```python
from build123d import *

# Parameters (mm, degrees)
F0_R     = 11.05
F0_R_2   = 1
F0_R_3   = 2
F1_DEPTH = 7


with BuildPart() as f1:
    # F0 (on Top) → F1 (new body)
    with BuildSketch(Plane.XY):
        with BuildLine():
            ThreePointArc((-8.1567643089, 17.1600465037), (0, 14.4299215496), (8.1567643089, 17.1600465037))
            ThreePointArc((8.1567643089, 17.1600465037), (12.1269669824, 21.9351575503), (13.55, 27.9799215496))
            ThreePointArc((13.55, 27.9799215496), (-6.0447639993, 40.106888532), (-8.1567643089, 17.1600465037))
        make_face()
        with Locations((0, 27.9799215496)):
            Circle(F0_R, mode=Mode.SUBTRACT)
        with BuildLine():
            ThreePointArc((37.7813228578, -13.9899607748), (31.7112023358, -2.6915581003), (18.9394183568, -1.5160581476))
            ThreePointArc((18.9394183568, -1.5160581476), (12.4966786365, -7.2149607748), (10.7826540478, -15.6439883561))
            ThreePointArc((10.7826540478, -15.6439883561), (25.0598871658, -27.5146042521), (37.7813228578, -13.9899607748))
        make_face()
        with Locations((24.2313228578, -13.9899607748)):
            Circle(F0_R, mode=Mode.SUBTRACT)
        with BuildLine():
            ThreePointArc((-18.9394183568, -1.5160581476), (-35.9659670791, -20.7649607748), (-10.7826540478, -15.6439883561))
            ThreePointArc((-10.7826540478, -15.6439883561), (-10.7066793805, -14.8185250827), (-10.6813228578, -13.9899607748))
            ThreePointArc((-10.6813228578, -13.9899607748), (-12.9329201833, -6.5100812968), (-18.9394183568, -1.5160581476))
        make_face()
        with Locations((-24.2313228578, -13.9899607748)):
            Circle(F0_R, mode=Mode.SUBTRACT)
        with BuildLine():
            ThreePointArc((4.7600365071, -12.6863924128), (11.1377958922, -7.7169944062), (13.55, 0))
            ThreePointArc((13.55, 0), (13.5004224782, 1.1580556593), (13.352052707, 2.3076369968))
            ThreePointArc((13.352052707, 2.3076369968), (11.7125847278, 6.8130653155), (8.6067198583, 10.4655087445))
            ThreePointArc((8.6067198583, 10.4655087445), (-0.0439952769, 13.549928576), (-8.6744986155, 10.4093983385))
            ThreePointArc((-8.6744986155, 10.4093983385), (-11.7565800048, 6.7368632605), (-13.3667563654, 2.2208836683))
            ThreePointArc((-13.3667563654, 2.2208836683), (-11.7125847278, -6.8130653155), (-4.6775540916, -12.7170353353))
            ThreePointArc((-4.6775540916, -12.7170353353), (0.0439952769, -13.549928576), (4.7600365071, -12.6863924128))
        make_face()
        Circle(F0_R, mode=Mode.SUBTRACT)
        with BuildLine():
            ThreePointArc((-8.7748548257, -16.8523565945), (-7.0337804641, -14.4799478416), (-4.6775540916, -12.7170353353))
            ThreePointArc((-4.6775540916, -12.7170353353), (-11.7125847278, -6.8130653155), (-13.3667563654, 2.2208836683))
            ThreePointArc((-13.3667563654, 2.2208836683), (-16.0640126782, 1.044247953), (-18.9869659815, 0.7036496412))
            ThreePointArc((-18.9869659815, 0.7036496412), (-18.9956424716, -0.4068993604), (-18.9394183568, -1.5160581476))
            ThreePointArc((-18.9394183568, -1.5160581476), (-12.9329201833, -6.5100812968), (-10.6813228578, -13.9899607748))
            ThreePointArc((-10.6813228578, -13.9899607748), (-10.7066793805, -14.8185250827), (-10.7826540478, -15.6439883561))
            ThreePointArc((-10.7826540478, -15.6439883561), (-9.7974015323, -16.2791560965), (-8.7748548257, -16.8523565945))
        make_face()
        with BuildLine():
            ThreePointArc((-8.6744986155, 10.4093983385), (-0.0439952769, 13.549928576), (8.6067198583, 10.4655087445))
            ThreePointArc((8.6067198583, 10.4655087445), (8.9363515943, 13.3897190895), (10.1028614554, 16.0913700602))
            ThreePointArc((10.1028614554, 16.0913700602), (9.1454360529, 16.6541586219), (8.1567643089, 17.1600465037))
            ThreePointArc((8.1567643089, 17.1600465037), (0, 14.4299215496), (-8.1567643089, 17.1600465037))
            ThreePointArc((-8.1567643089, 17.1600465037), (-9.1994619657, 16.6243766663), (-10.2071415116, 16.0254254908))
            ThreePointArc((-10.2071415116, 16.0254254908), (-9.0231124442, 13.3314064874), (-8.6744986155, 10.4093983385))
        make_face()
        with BuildLine():
            ThreePointArc((13.352052707, 2.3076369968), (13.5004224782, 1.1580556593), (13.55, 0))
            ThreePointArc((13.55, 0), (11.1377958922, -7.7169944062), (4.7600365071, -12.6863924128))
            ThreePointArc((4.7600365071, -12.6863924128), (7.1276610839, -14.4339670425), (8.8841045261, -16.7950197013))
            ThreePointArc((8.8841045261, -16.7950197013), (9.8502064187, -16.2472592614), (10.7826540478, -15.6439883561))
            ThreePointArc((10.7826540478, -15.6439883561), (12.4966786365, -7.2149607748), (18.9394183568, -1.5160581476))
            ThreePointArc((18.9394183568, -1.5160581476), (18.9968634979, -0.3452205697), (18.9819963373, 0.8269311037))
            ThreePointArc((18.9819963373, 0.8269311037), (16.0568929083, 1.1485413542), (13.352052707, 2.3076369968))
        make_face()
        with BuildLine():
            ThreePointArc((8.6067198583, 10.4655087445), (11.7125847278, 6.8130653155), (13.352052707, 2.3076369968))
            ThreePointArc((13.352052707, 2.3076369968), (16.0568929083, 1.1485413542), (18.9819963373, 0.8269311037))
            ThreePointArc((18.9819963373, 0.8269311037), (23.4304012279, 2.0634206387), (26.8491945381, 5.1664940737))
            ThreePointArc((26.8491945381, 5.1664940737), (28.2136339107, 8.0652639574), (28.5913217984, 11.246759439))
            ThreePointArc((28.5913217984, 11.246759439), (27.2444210774, 15.8477419457), (23.9108601236, 19.2931088268))
            ThreePointArc((23.9108601236, 19.2931088268), (20.9586164714, 20.5376244184), (17.7643170713, 20.7846324805))
            ThreePointArc((17.7643170713, 20.7846324805), (13.3768238274, 19.3468858147), (10.1028614554, 16.0913700602))
            ThreePointArc((10.1028614554, 16.0913700602), (8.9363515943, 13.3897190895), (8.6067198583, 10.4655087445))
        make_face()
        with BuildLine():
            ThreePointArc((12.9505363993, 11.1563030517), (13.5264237307, 11.5666124247), (13.9367331037, 10.9907250933))
            ThreePointArc((13.9367331037, 10.9907250933), (14.5872544025, 8.309022028), (16.9762482984, 6.9279291798))
            ThreePointArc((16.9762482984, 6.9279291798), (17.4128850212, 6.3717382302), (16.8566940716, 5.9351015075))
            ThreePointArc((16.8566940716, 5.9351015075), (13.7865377349, 7.7099787756), (12.9505363993, 11.1563030517))
        make_face(mode=Mode.SUBTRACT)
        with Locations((18.6004471086, 10.8196494619)):
            Circle(F0_R_2, mode=Mode.SUBTRACT)
        with Locations((23.5651301856, 10.2264193675)):
            Circle(F0_R_3, mode=Mode.SUBTRACT)
        with Locations((20.539148591, 15.4284927617)):
            Circle(F0_R_3, mode=Mode.SUBTRACT)
        with BuildLine():
            ThreePointArc((28.5913217984, 11.246759439), (28.2136339107, 8.0652639574), (26.8491945381, 5.1664940737))
            ThreePointArc((26.8491945381, 5.1664940737), (30.4593772075, 4.9963032192), (33.5974550448, 6.789303866))
            ThreePointArc((33.5974550448, 6.789303866), (32.1424199084, 10.1950675609), (28.5913217984, 11.246759439))
        make_face()
        with BuildLine():
            ThreePointArc((22.5110596529, 25.8483234616), (19.4011285413, 24.00693477), (17.7643170713, 20.7846324805))
            ThreePointArc((17.7643170713, 20.7846324805), (20.9586164714, 20.5376244184), (23.9108601236, 19.2931088268))
            ThreePointArc((23.9108601236, 19.2931088268), (24.7522139126, 22.8998355139), (22.5110596529, 25.8483234616))
        make_face()
        with BuildLine():
            ThreePointArc((-13.3667563654, 2.2208836683), (-11.7565800048, 6.7368632605), (-8.6744986155, 10.4093983385))
            ThreePointArc((-8.6744986155, 10.4093983385), (-9.0231124442, 13.3314064874), (-10.2071415116, 16.0254254908))
            ThreePointArc((-10.2071415116, 16.0254254908), (-13.5021753057, 19.2596123649), (-17.8989123854, 20.6688375043))
            ThreePointArc((-17.8989123854, 20.6688375043), (-21.0915404306, 20.401091721), (-24.0356402836, 19.1374312857))
            ThreePointArc((-24.0356402836, 19.1374312857), (-27.3467576563, 15.6704897916), (-28.6637524238, 11.06085788))
            ThreePointArc((-28.6637524238, 11.06085788), (-28.2654127155, 7.8818820832), (-26.8821782721, 4.9920336244))
            ThreePointArc((-26.8821782721, 4.9920336244), (-23.4433065133, 1.9112263491), (-18.9869659815, 0.7036496412))
            ThreePointArc((-18.9869659815, 0.7036496412), (-16.0640126782, 1.044247953), (-13.3667563654, 2.2208836683))
        make_face()
        with Locations((-23.6310409692, 10.0731780711)):
            Circle(F0_R_3, mode=Mode.SUBTRACT)
        with Locations((-20.6389040547, 15.2947917005)):
            Circle(F0_R_3, mode=Mode.SUBTRACT)
        with BuildLine():
            ThreePointArc((-13.5682957153, 11.6307745361), (-13.5703063498, 8.0845025208), (-16.1369100547, 5.6373419886))
            ThreePointArc((-16.1369100547, 5.6373419886), (-16.7801920608, 5.9309203608), (-16.4866136886, 6.5742023669))
            ThreePointArc((-16.4866136886, 6.5742023669), (-14.4894513581, 8.47842187), (-14.4878868145, 11.2378976975))
            ThreePointArc((-14.4878868145, 11.2378976975), (-14.2245296842, 11.8941316664), (-13.5682957153, 11.6307745361))
        make_face(mode=Mode.SUBTRACT)
        with Locations((-18.6703148483, 10.6986349868)):
            Circle(F0_R_2, mode=Mode.SUBTRACT)
        with BuildLine():
            ThreePointArc((-24.0356402836, 19.1374312857), (-21.0915404306, 20.401091721), (-17.8989123854, 20.6688375043))
            ThreePointArc((-17.8989123854, 20.6688375043), (-19.5566141165, 23.8804428355), (-22.6784371444, 25.7015976383))
            ThreePointArc((-22.6784371444, 25.7015976383), (-24.9003974552, 22.7386183993), (-24.0356402836, 19.1374312857))
        make_face()
        with BuildLine():
            ThreePointArc((-33.6408345895, 6.5709877947), (-30.4911796484, 4.7984027938), (-26.8821782721, 4.9920336244))
            ThreePointArc((-26.8821782721, 4.9920336244), (-28.2654127155, 7.8818820832), (-28.6637524238, 11.06085788))
            ThreePointArc((-28.6637524238, 11.06085788), (-32.2079462538, 9.9861282912), (-33.6408345895, 6.5709877947))
        make_face()
        with BuildLine():
            ThreePointArc((8.8841045261, -16.7950197013), (7.1276610839, -14.4339670425), (4.7600365071, -12.6863924128))
            ThreePointArc((4.7600365071, -12.6863924128), (0.0439952769, -13.549928576), (-4.6775540916, -12.7170353353))
            ThreePointArc((-4.6775540916, -12.7170353353), (-7.0337804641, -14.4799478416), (-8.7748548257, -16.8523565945))
            ThreePointArc((-8.7748548257, -16.8523565945), (-9.9282259222, -21.3230330036), (-8.9502821528, -25.835331578))
            ThreePointArc((-8.9502821528, -25.835331578), (-7.12209348, -28.4663556784), (-4.5556815148, -30.3841907247))
            ThreePointArc((-4.5556815148, -30.3841907247), (0.1023365788, -31.5182317373), (4.7528923002, -30.3539667068))
            ThreePointArc((4.7528923002, -30.3539667068), (7.3067962441, -28.4195065016), (9.1178612008, -25.7766661049))
            ThreePointArc((9.1178612008, -25.7766661049), (10.0664826859, -21.2581121638), (8.8841045261, -16.7950197013))
        make_face()
        with Locations((-2.9262261308, -25.5212110679)):
            Circle(F0_R_3, mode=Mode.SUBTRACT)
        with BuildLine():
            ThreePointArc((3.1863736554, -16.7936450403), (3.2537683301, -17.4975327855), (2.549880585, -17.5649274602))
            ThreePointArc((2.549880585, -17.5649274602), (-0.0978030444, -16.787443898), (-2.4883614839, -18.1658268773))
            ThreePointArc((-2.4883614839, -18.1658268773), (-3.1883553369, -18.2658698966), (-3.2883983563, -17.5658760436))
            ThreePointArc((-3.2883983563, -17.5658760436), (-0.2162313851, -15.7944812964), (3.1863736554, -16.7936450403))
        make_face(mode=Mode.SUBTRACT)
        with Locations((3.0918923782, -25.5016708328)):
            Circle(F0_R_3, mode=Mode.SUBTRACT)
        with Locations((0.0698677398, -21.5182844487)):
            Circle(F0_R_2, mode=Mode.SUBTRACT)
        with BuildLine():
            ThreePointArc((-4.5556815148, -30.3841907247), (-7.12209348, -28.4663556784), (-8.9502821528, -25.835331578))
            ThreePointArc((-8.9502821528, -25.835331578), (-10.9027630909, -28.8767460547), (-10.9190179004, -32.4909015044))
            ThreePointArc((-10.9190179004, -32.4909015044), (-7.2420224532, -32.9336859602), (-4.5556815148, -30.3841907247))
        make_face()
        with BuildLine():
            ThreePointArc((11.1297749366, -32.4193112564), (11.0900511072, -28.8053375638), (9.1178612008, -25.7766661049))
            ThreePointArc((9.1178612008, -25.7766661049), (7.3067962441, -28.4195065016), (4.7528923002, -30.3539667068))
            ThreePointArc((4.7528923002, -30.3539667068), (7.4557323412, -32.8859638051), (11.1297749366, -32.4193112564))
        make_face()
    extrude(amount=F1_DEPTH)


solid = f1.part
```
CAD build for the part. Positions are in the model's coordinates, mm. Coordinates: 2 decimals unless noted, no trailing zeros. Order: outer loops, then holes, each group sorted by start corner. A loop starts at its lowest first (then second) coordinate and runs counter-clockwise, first axis right, second up.
(1) Drill centre lines: L1, parallel to X at y = -13.5, z = 3.75; L2, parallel to Y at x = 0, z = 3.5; L3, parallel to Y at x = -8.5, z = 1.75. Where is each one in solid material? Low to high.
Solution:
L1: x = -37.77 to -35.27, -13.19 to 13.19, 35.27 to 37.77
L2: y = -31.52 to -22.52, -20.52 to -16.78, -15.77 to -11.05, 11.05 to 16.93, 39.03 to 41.53
L3: y = -33.15 to -7.06, 7.06 to 16.99, 17.43 to 20.92, 35.04 to 38.53
(2) Saw through at C-C, the plane x = 0. Write the cut outline in (y, z), and give its area (3 significant figures).
Solution:
outline: (-31.52, 0) - (-22.52, 0) - (-22.52, 7) - (-31.52, 7) - close; (-20.52, 0) - (-16.78, 0) - (-16.78, 7) - (-20.52, 7) - close; (-15.77, 0) - (-11.05, 0) - (-11.05, 7) - (-15.77, 7) - close; (11.05, 0) - (16.93, 0) - (16.93, 7) - (11.05, 7) - close; (39.03, 0) - (41.53, 0) - (41.53, 7) - (39.03, 7) - close
area: 181 mm2
(3) Mould opens along Y. For faces 1 (the face through (34.77, -10.67, 3.45)), 2 (the face through (-11.4, 1.6, 7)), 3 (the face through (19.436, 24.044, 3.451)) say: released by +Y, released by -Y, zero draft, split by the parting line, or undercut.
Solution:
face 1: undercut
face 2: zero draft
face 3: released by +Y
(4) Saw through at D-D, the plane z = 5.75. Count the separate pieces of the cut face and the enclosed holes in it, and give its area (3 significant figures).
Solution:
separate pieces: 1
enclosed holes: 16
area: 1,910 mm2
(5) Saw through at A-A, the plane y = 29. Write the cut outline in (x, z), and give its area (3 significant figures).
Solution:
outline: (-13.51, 0) - (-11, 0) - (-11, 7) - (-13.51, 7) - close; (11, 0) - (13.51, 0) - (13.51, 7) - (11, 7) - close
area: 35.1 mm2
(6) Saw through at B-B, the plane x = -32.5. Write the cut outline in (y, z).
Solution:
outline: (-24.72, 0) - (-21.32, 0) - (-21.32, 7) - (-24.72, 7) - close; (-6.66, 0) - (-3.26, 0) - (-3.26, 7) - (-6.66, 7) - close; (5.64, 0) - (9.7, 0) - (9.7, 7) - (5.64, 7) - close
(7) Pin check, flat tips, straight feed: pin 1 Ø1 at (x, z) = (18.5, 4) entering from +Y; pin 2 Ø3 at (y, z) = (-0.5, 3.5) entering from -X; pin 3 Ø1 at (x, z) = (26.5, 3) entering from +Y. Stop position of each tip, or through.
Solution:
pin 1: stops at y = 23.54
pin 2: stops at x = -30.54
pin 3: stops at y = 17.55
